```python
from build123d import *

# Parameters (mm, degrees)
SKETCH_1_W      = 22.4
SKETCH_1_H      = 12.5
EXTRUDE_1_DEPTH = 16.1
SKETCH_2_W      = 31.8
SKETCH_2_H      = 12.5
SKETCH_2_R      = 1.5
EXTRUDE_2_DEPTH = 3
SKETCH_3_W      = 22.4
SKETCH_3_H      = 12.5
EXTRUDE_3_DEPTH = 22.8
SKETCH_4_R      = 5
EXTRUDE_4_DEPTH = 5
SKETCH_5_R      = 2
EXTRUDE_5_DEPTH = 30.9


with BuildPart() as part:
    # 草图1 → 凸台-拉伸1 (new body)
    with BuildSketch(Plane(origin=(0, 0, 0), x_dir=(1, 0, 0), z_dir=(0, 1, 0))):
        Rectangle(SKETCH_1_W, SKETCH_1_H)
    extrude(amount=EXTRUDE_1_DEPTH)

    # 草图2 → 凸台-拉伸2 (add)
    with BuildSketch(Plane(origin=(0, 16.1, 0), x_dir=(1, 0, 0), z_dir=(0, 1, 0))):
        Rectangle(SKETCH_2_W, SKETCH_2_H)
        with Locations((13.85, 0)):
            Circle(SKETCH_2_R, mode=Mode.SUBTRACT)
        with Locations((-13.85, 0)):
            Circle(SKETCH_2_R, mode=Mode.SUBTRACT)
    extrude(amount=EXTRUDE_2_DEPTH)

    # 草图3 → 凸台-拉伸3 (add)
    with BuildSketch(Plane.XZ):
        Rectangle(SKETCH_3_W, SKETCH_3_H)
    extrude(amount=-EXTRUDE_3_DEPTH)

    # 草图4 → 凸台-拉伸4 (add)
    with BuildSketch(Plane(origin=(0, 22.8, 0), x_dir=(1, 0, 0), z_dir=(0, 1, 0))):
        with Locations((6.2, 0)):
            Circle(SKETCH_4_R)
    extrude(amount=EXTRUDE_4_DEPTH)

    # 草图5 → 凸台-拉伸5 (add)
    with BuildSketch(Plane.XZ):
        with Locations((6.2, 0)):
            Circle(SKETCH_5_R)
    extrude(amount=-EXTRUDE_5_DEPTH)


solid = part.part
```
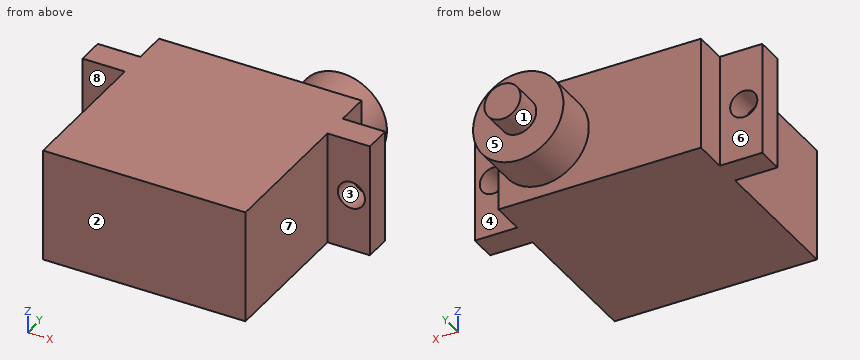
The listing builds one solid part. Answer for the finished solid, in the listing's coordinates (mm). Face numbers are marked on the shaded views. A direction names the side the tool comes from. Coordinates: 2 decimals unless noted, no trailing zeros. Loops run counter-clockwise (first coordinate to the right, second up) from the corner with the lowest first, then second, coordinate; pieces in that order, holes last. Notation, with made-up numbers: (57.5, 35.25) -> (61.5, 35.25) arc R8 ccw to (61.5, 47.25) -> close; hole circle Ø5 at (7.25, 15). An arc over 180 degrees is marked (long way). Use one line per item in the form item = value. Start each with the question number.
Item 1: The part is cut by section A-A on x = -13.85. Determine the outline of the cut face in (y, z).
Item 2: The mould has two halves that part along X. Classify the marked faces 1, 2 and 3: released by +X, released by -X, zero draft, split by the parting line, or undercut.
Item 3: The part is cut by section C-C on x = 6.2. Determine the outline of the cut face in (y, z).
Item 4: Consider L1, parallel to X at y = 18.4, z = 0; L2, parallel to Z at x = 13.85, y = 17; L3, parallel to Y at x = 1.5, z = 4.25. Determine where each line is inside the solid, lowest interval first. Write a range as [from, to].
Item 5: The part is cut by section D-D on y = 13. Determine the outline of the cut face in (x, z).
Item 6: A tool of negligible diameter and unlimited length cuts with its end or side. For the marked faces 4, 5, 6, 7 and 8, from which of +Z, -Z, +X, -X, +Y, -Y can it reach the whole face along a straight path? Write none if from no direction.
Item 7: The part is cut by section B-B on z = 1. Determine the outline of the cut face in (x, y), then the cut area to 3 significant figures.
Item 8: Flat-ended cylindrical pins translate along their axes: pin 1 Ø3 at (y, z) = (4.5, -5) entering from -X; pin 2 Ø1.5 at (y, z) = (26, -1.5) entering from +X; pin 3 Ø2.5 at (x, z) = (-12.5, -1.5) entering from +Y; pin 4 Ø2.5 at (x, z) = (-13.85, 0) entering from -Y. Find the tip coordinate at first contact, or state that the pin passes through.
Answer key:
q1.outline = (16.1, -6.25) -> (19.1, -6.25) -> (19.1, -1.5) -> (16.1, -1.5) -> close; (16.1, 1.5) -> (19.1, 1.5) -> (19.1, 6.25) -> (16.1, 6.25) -> close
q2.face_1 = split by the parting line
q2.face_2 = zero draft
q2.face_3 = undercut
q3.outline = (0, -6.25) -> (22.8, -6.25) -> (22.8, -5) -> (27.8, -5) -> (27.8, -2) -> (30.9, -2) -> (30.9, 2) -> (27.8, 2) -> (27.8, 5) -> (22.8, 5) -> (22.8, 6.25) -> (0, 6.25) -> close
q4.L1 = [-15.9, -15.35], [-12.35, 12.35], [15.35, 15.9]
q4.L2 = [-6.25, -1.5], [1.5, 6.25]
q4.L3 = [0, 22.8]
q5.outline = (-11.2, -6.25) -> (11.2, -6.25) -> (11.2, 6.25) -> (-11.2, 6.25) -> close
q6.face_4 = +Z, -Z, +X, +Y
q6.face_5 = +Y
q6.face_6 = +Z, -Z, -X, +Y
q6.face_7 = +Z, -Z, +X, -Y
q6.face_8 = +Z, -Z, -X, -Y
q7.outline = (-15.9, 16.1) -> (-14.97, 16.1) -> (-14.97, 19.1) -> (-15.9, 19.1) -> close; (-12.73, 16.1) -> (-11.2, 16.1) -> (-11.2, 0) -> (11.2, 0) -> (11.2, 16.1) -> (12.73, 16.1) -> (12.73, 19.1) -> (11.2, 19.1) -> (11.2, 22.8) -> (11.1, 22.8) -> (11.1, 27.8) -> (7.93, 27.8) -> (7.93, 30.9) -> (4.47, 30.9) -> (4.47, 27.8) -> (1.3, 27.8) -> (1.3, 22.8) -> (-11.2, 22.8) -> (-11.2, 19.1) -> (-12.73, 19.1) -> close; (14.97, 16.1) -> (15.9, 16.1) -> (15.9, 19.1) -> (14.97, 19.1) -> close
q7.area = 585 mm2
q8.pin_1 = -11.2
q8.pin_2 = 11.14
q8.pin_3 = 19.1
q8.pin_4 = through
